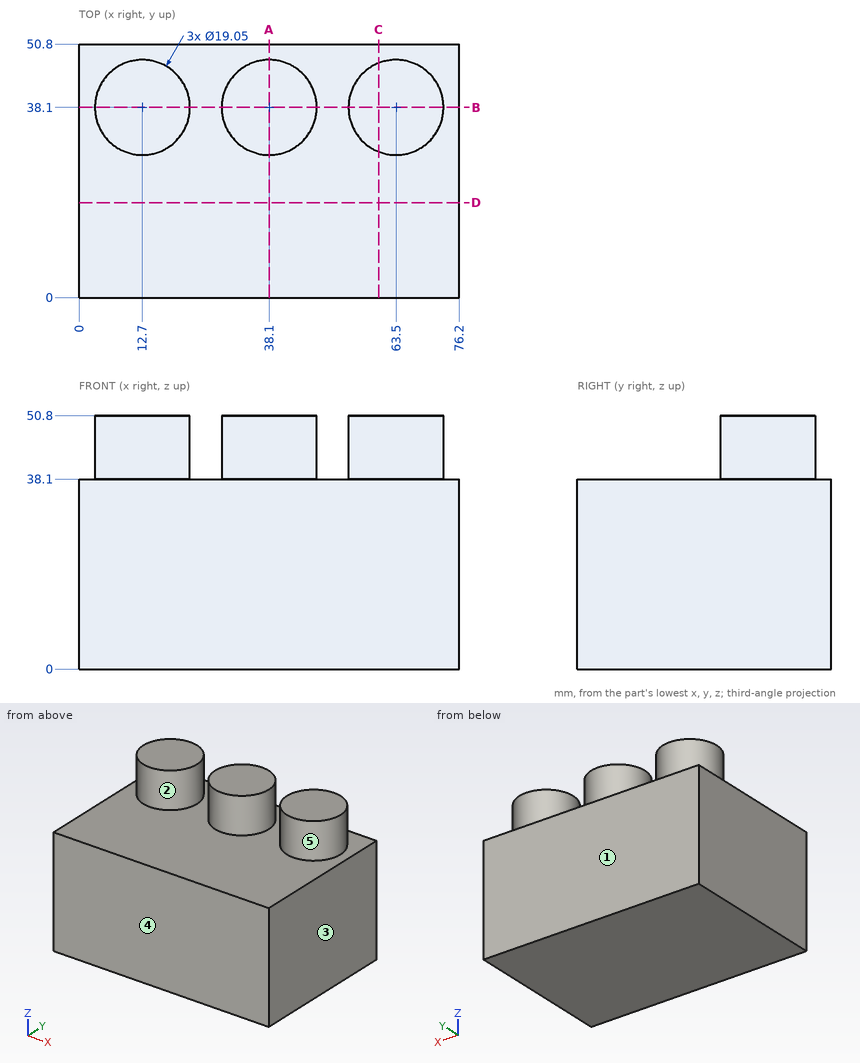
Answer from the drawing. Dimensions are ordinates in mm from the lowest x, y and z of the part. A direction names the side the tool comes from. Coordinates: 2 decimals unless noted, no trailing zeros. Order: outer loops, then holes, each group sorted by start corner. A loop starts at its lowest first (then second) coordinate and runs counter-clockwise, first axis right, second up. Notation, with made-up numbers: (15, -1) - (48, -1) arc R34 ccw to (48, 35) - close; hole circle Ø6 at (66, -1). An arc over 180 degrees is marked (long way). Put each result on its own line as item: value. Start each with the question number.
1) For a pull along X with two mould halves and no side action, classify the marked faces 1, 2 and 3 as released by +X, released by -X, zero draft, split by the parting line, or undercut.
2) Find section C-C (x = 60). Give the vertices of the cut face in (y, z), plus the area to 3 significant figures.
3) Find section A-A (x = 38.1). Give the vertices of the cut face in (y, z) (3 decimals).
4) Find the intervals of material crossed by line 1 (X direction, y = 43.5, z = 47.5); line 2 (Z direction, x = 4, y = 25); line 3 (Y direction, x = 7.5, z = 48), in increasing order. Write a range as from..to.
5) Find section D-D (y = 19). Give the vertices of the cut face in (x, z).
6) Find section B-B (y = 38.1). Give the vertices of the cut face in (x, z) (3 decimals).
7) Flat-ended cylindrical pins translate along their axes: pin 1 (1 mm diameter, centred on x = 51, y = 41, fed in from +Z); pin 2 (5 mm diameter, centred on y = 27.5, z = 44, fed in from +X). Find the tip coordinate at first contact, or state that the pin passes through.
8) For the marked faces 4 and 5, determine the directions among +Z, -Z, +X, -X, +Y, -Y from which every point of the face is accessible in a straight line to the end or side of a thin tool.
Results list:
1. face 1: zero draft
1. face 2: undercut
1. face 3: released by +X
2. outline: (0, 0) - (50.8, 0) - (50.8, 38.1) - (46.96, 38.1) - (46.96, 50.8) - (29.24, 50.8) - (29.24, 38.1) - (0, 38.1) - close
2. area: 2,160 mm^2
3. outline: (0, 0) - (50.8, 0) - (50.8, 38.1) - (47.625, 38.1) - (47.625, 50.8) - (28.575, 50.8) - (28.575, 38.1) - (0, 38.1) - close
4. line 1: x = 4.85..20.55, 30.25..45.95, 55.65..71.35
4. line 2: z = 0..38.1
4. line 3: y = 30.12..46.08
5. outline: (0, 0) - (76.2, 0) - (76.2, 38.1) - (0, 38.1) - close
6. outline: (0, 0) - (76.2, 0) - (76.2, 38.1) - (73.025, 38.1) - (73.025, 50.8) - (53.975, 50.8) - (53.975, 38.1) - (47.625, 38.1) - (47.625, 50.8) - (28.575, 50.8) - (28.575, 38.1) - (22.225, 38.1) - (22.225, 50.8) - (3.175, 50.8) - (3.175, 38.1) - (0, 38.1) - close
7. pin 1: stops at z = 38.1
7. pin 2: stops at x = 68.51
8. face 4: +Z, -Z, +X, -X, -Y
8. face 5: +Z
